Input: part model. Units: mm. Frame: model coordinates. A direction names the side the tool comes from. Coordinates: 2 decimals unless noted, no trailing zeros. Loops run counter-clockwise (first coordinate to the right, second up) from the corner with the lowest first, then second, coordinate; pieces in that order, holes last.
(1) Section B-B, the plane x = -127.5. Return loops of the section in (y, z), then the cut area to 4 significant figures.
(2) Mould query, pull axis Y, two halves, no side actions, for faces 4 (the face through (-1, -234.76, 123)), 5 (the face through (-212, 178, 25)), 6 (the face through (-1, 18, 25)), 7 (the face through (-1, 240.24, 136)). Classes: released by +Y, released by -Y, zero draft, split by the parting line, or undercut.
(3) Line query: L1, parallel to X at y = 182.5, z = 138; L2, parallel to Y at x = 5.5, z = 41; L3, parallel to Z at x = -17.5, y = 144.5. Output: solid intervals per line, ascending.
(4) Set-up query: faces 1 (the face through (-1, -209.76, 136)), 2 (the face through (-212, 178, 29)), 3 (the face through (-177, 35, 250)). Return all of +Z, -Z, +X, -X, +Y, -Y with unobstructed straight access to the full face (end or side cutting, diameter ignored); none if empty.
(5) Section C-C, the plane y = 18. Return loops of the section in (x, z), then the cut area to 4 significant figures.
(6) Contact query for flat-ended pins moving along their axis: P1, Ø2, axis at x = -219, z = 26, coming from the +Y side; P2, Ø8, axis at x = -209, y = 179, coming from the +Z side; P3, Ø5, axis at y = 130, z = 188, coming from the -X side. Output: stop coordinate, or through.
(7) Section A-A, the plane z = 186.5. Return loops of the section in (x, y).
```python
from build123d import *

# Parameters (mm, degrees)
F0_W     = 400
F0_H     = 500
F1_DEPTH = 250
F2_T     = -25
F3_W     = 59.44657
F3_H     = 26.272267
F4_DEPTH = 4
F5_R     = 5
F6_R     = 7.658555
F7_DEPTH = 25


with BuildPart() as f1:
    # F0 (on Top) → F1 (new body)
    with BuildSketch(Plane.XY):
        with Locations((1.677677, 15.239688)):
            Rectangle(F0_W, F0_H)
    extrude(amount=F1_DEPTH)

    # F2
    f2_openings = [f1.faces().sort_by_distance(p)[0] for p in [
        (1.677677, 15.239688, 250),
    ]]
    offset(amount=F2_T, openings=f2_openings)

    # F3 (on face) → F4 (join)
    with BuildSketch(Plane.XY.offset(25)):
        with Locations((-203.045608, 174.877093)):
            Rectangle(F3_W, F3_H)
    extrude(amount=F4_DEPTH)

    # F5
    f5_edges = [f1.edges().sort_by_distance(p)[0] for p in [
        (-232.768893, 161.740959, 27),
        (-232.768893, 188.013226, 27),
    ]]
    fillet(f5_edges, radius=F5_R)

    # F6 (on face) → F7 (cut)
    with BuildSketch(Plane.XY.offset(29)):
        with Locations((-219.607025, 174.877092)):
            Circle(F6_R)
    extrude(amount=-F7_DEPTH, mode=Mode.SUBTRACT)


solid = f1.part
```
Report:
1. outline: (-234.76, 0) - (265.24, 0) - (265.24, 250) - (240.24, 250) - (240.24, 25) - (-209.76, 25) - (-209.76, 250) - (-234.76, 250) - close
1. area: 23,750 mm2
2. face 4: released by -Y
2. face 5: zero draft
2. face 6: undercut
2. face 7: undercut
3. L1: x = -198.32 to -173.32, 176.68 to 201.68
3. L2: y = -234.76 to -209.76, 240.24 to 265.24
3. L3: z = 0 to 25
4. face 1: +Z
4. face 2: +Z, -X, +Y, -Y
4. face 3: +Z, +X, -X, +Y, -Y
5. outline: (-198.32, 0) - (201.68, 0) - (201.68, 250) - (176.68, 250) - (176.68, 25) - (-173.32, 25) - (-173.32, 250) - (-198.32, 250) - close
5. area: 21,250 mm2
6. P1: stops at y = 188.01
6. P2: stops at z = 29
6. P3: stops at x = -198.32
7. outline: (-198.32, -234.76) - (201.68, -234.76) - (201.68, 265.24) - (-198.32, 265.24) - close; hole (-173.32, -209.76) - (176.68, -209.76) - (176.68, 240.24) - (-173.32, 240.24) - close
